Model file for the job. Use its own axes, mm. A direction names the side the tool comes from. Coordinates: 2 decimals unless noted, no trailing zeros. Order: outer loops, then holes, each group sorted by start corner. A loop starts at its lowest first (then second) coordinate and runs counter-clockwise, first axis right, second up. Notation, with made-up numbers: M 10.25,1.5 L 33.25,1.5 A11 cw 33.25,10.5 Z; hole C 8.5,7.25 d8. An arc over 180 degrees is marked long. Return JSON: item names as keys, results as strings.
```python
from build123d import *

# Parameters (mm, degrees)
SKETCH_W        = 150
SKETCH_H        = 120
SKETCH_R        = 4.5
SKETCH_R_2      = 1.75
SKETCH_R_3      = 2
PAD_DEPTH       = 3
PAD001_DEPTH    = 7
SKETCH003_R     = 1.75
POCKET_DEPTH    = 5
SKETCH002_R     = 1.75
POCKET001_DEPTH = 5
SKETCH004_R     = 1.75
POCKET002_DEPTH = 5


with BuildPart() as part:
    # Sketch → Pad (new body)
    with BuildSketch(Plane.XY):
        with Locations((75, 60)):
            Rectangle(SKETCH_W, SKETCH_H)
        with Locations((20, 90)):
            Circle(SKETCH_R, mode=Mode.SUBTRACT)
        with Locations((13.75, 96.25)):
            Circle(SKETCH_R_2, mode=Mode.SUBTRACT)
        with Locations((26.25, 96.25)):
            Circle(SKETCH_R_2, mode=Mode.SUBTRACT)
        with Locations((13.75, 83.75)):
            Circle(SKETCH_R_2, mode=Mode.SUBTRACT)
        with Locations((26.25, 83.75)):
            Circle(SKETCH_R_2, mode=Mode.SUBTRACT)
        with Locations((4, 116)):
            Circle(SKETCH_R_2, mode=Mode.SUBTRACT)
        with Locations((4, 4)):
            Circle(SKETCH_R_2, mode=Mode.SUBTRACT)
        with Locations((45, 104)):
            Circle(SKETCH_R_3, mode=Mode.SUBTRACT)
        with Locations((136.6, 104)):
            Circle(SKETCH_R_3, mode=Mode.SUBTRACT)
        with Locations((45, 12)):
            Circle(SKETCH_R_3, mode=Mode.SUBTRACT)
        with Locations((136.6, 12)):
            Circle(SKETCH_R_3, mode=Mode.SUBTRACT)
        Polygon((49, 108), (110, 108), (110, 115), (120, 115), (120, 108), (132.6, 108), (132.6, 100), (140.6, 100), (140.6, 16), (132.6, 16), (132.6, 8), (49, 8), (49, 16), (41, 16), (41, 29), (26, 29), (26, 52), (41, 52), (41, 100), (49, 100), align=None, mode=Mode.SUBTRACT)
    extrude(amount=-PAD_DEPTH)

    # Sketch001 (on DatumPlane) → Pad001 (join)
    with BuildSketch(Plane.XY.offset(-3)):
        Polygon((15, 117), (15, 120), (150, 120), (150, 0), (15, 0), (15, 3), (147, 3), (147, 117), align=None)
    extrude(amount=-PAD001_DEPTH)

    # Sketch003 (on DatumPlane) → Pocket (cut)
    with BuildSketch(Plane.XZ.offset(-120)):
        with Locations((25, -6.5)):
            Circle(SKETCH003_R)
        with Locations((75, -6.5)):
            Circle(SKETCH003_R)
        with Locations((125, -6.5)):
            Circle(SKETCH003_R)
    extrude(amount=POCKET_DEPTH, mode=Mode.SUBTRACT)

    # Sketch002 → Pocket001 (cut)
    with BuildSketch(Plane.XZ):
        with Locations((25, -6.5)):
            Circle(SKETCH002_R)
        with Locations((75, -6.5)):
            Circle(SKETCH002_R)
        with Locations((125, -6.5)):
            Circle(SKETCH002_R)
    extrude(amount=-POCKET001_DEPTH, mode=Mode.SUBTRACT)

    # Sketch004 (on DatumPlane) → Pocket002 (cut, symmetric)
    with BuildSketch(Plane.YZ.offset(150)):
        with Locations((10, -6.5)):
            Circle(SKETCH004_R)
        with Locations((110, -6.156497)):
            Circle(SKETCH004_R)
        with Locations((60, -6.5)):
            Circle(SKETCH004_R)
    extrude(amount=POCKET002_DEPTH, both=True, mode=Mode.SUBTRACT)


solid = part.part
```
Item 1: Saw through at A-A (y = 67). Write the cut outline in (x, z), and give its area (3 significant figures).
Check result:
{"outline": "M 0,-3 L 41,-3 L 41,0 L 0,0 Z; M 140.6,-3 L 147,-3 L 147,-10 L 150,-10 L 150,0 L 140.6,0 Z", "area": "172 mm2"}
Item 2: Pull direction Y, two halves, no side cores. Call faces 1 (the cylindrical face through (23.61, 1.48, -7.56)), 2 (the flat face through (120, 112, -1)), 3 (the flat face through (74, 120, -4)): +Y half, -Y half, draft (parallel to the pull), parting line (faces both ways), or undercut.
Check result:
{"face 1": "draft", "face 2": "undercut", "face 3": "+Y half"}
Item 3: Wall check: line 1 (Y direction, x = 13.75, z = -1); line 2 (X direction, y = 83.5, z = -0.25); line 3 (Y direction, x = 59.5, z = -2.5). Give the ranges that are in metal, low to high.
Check result:
{"line 1": "y = 0 to 82, 85.5 to 94.5, 98 to 120", "line 2": "x = 0 to 12.02, 15.48 to 24.52, 27.98 to 41, 140.6 to 150", "line 3": "y = 0 to 8, 108 to 120"}
Item 4: Saw through at D-D (x = 71). Write the cut outline in (y, z), and give its area (3 significant figures).
Check result:
{"outline": "M 0,-10 L 3,-10 L 3,-3 L 8,-3 L 8,0 L 0,0 Z; M 108,-3 L 117,-3 L 117,-10 L 120,-10 L 120,0 L 108,0 Z", "area": "102 mm2"}
Item 5: Drop flat-ended pins along their axis: pin 1 Ø10 at (x, y) = (26, 25.5) entering from -Z; pin 2 Ø2.5 at (y, z) = (119, -5.5) entering from -X; pin 3 Ø1.5 at (y, z) = (60.5, -5) entering from -X; pin 4 Ø2 at (x, y) = (4, 4) entering from +Z. Give the stop position or say it passes through.
Check result:
{"pin 1": "stops at z = -3", "pin 2": "stops at x = 15", "pin 3": "stops at x = 147", "pin 4": "passes through"}
Item 6: Saw through at C-C (y = 96.25). Write the cut outline in (x, z), and give its area (3 significant figures).
Check result:
{"outline": "M 0,-3 L 12,-3 L 12,0 L 0,0 Z; M 15.5,-3 L 24.5,-3 L 24.5,0 L 15.5,0 Z; M 28,-3 L 41,-3 L 41,0 L 28,0 Z; M 140.6,-3 L 147,-3 L 147,-10 L 150,-10 L 150,0 L 140.6,0 Z", "area": "151 mm2"}
Item 7: Saw through at B-B (x = 38). Write the cut outline in (y, z).
Check result:
{"outline": "M 0,-10 L 3,-10 L 3,-3 L 29,-3 L 29,0 L 0,0 Z; M 52,-3 L 117,-3 L 117,-10 L 120,-10 L 120,0 L 52,0 Z"}
Item 8: 3-axis set-ups, long thin cutter, end or side, ignore diameter. For faces 4 (the flat face through (45, 16, -1)), 5 (the flat face through (80, 3, -6)), 6 (the flat face through (15, 1, -6)), 7 (the cylindrical face through (148.52, 10.81, -8.05)), 8 (the flat face through (150, 61, -4)): which of +Z, -Z, +X, -X, +Y, -Y reach the whole face in a straight line?
Check result:
{"face 4": "+Z, -Z", "face 5": "-Z, -X", "face 6": "-Z, -X, +Y, -Y", "face 7": "+X, -X", "face 8": "+Z, -Z, +X, +Y, -Y"}
